Study the drawing (mm; zero at the part's minimum x, y, z) and answer. A direction names the side the tool comes from. Round coordinates to 2 decimals unless told otherwise and drop trailing zeros. Write each loop counter-clockwise with the first axis right and the second up, starting at its lowest first coordinate (ties: lowest second). Pieces come first, ordered by that corner, then holes. Notation, with made-up numbers: (9.5, -15.5) -> (41.5, -15.5) arc R17 ccw to (41.5, 3.5) -> close; hole circle Ø7 at (75, -15.5). An arc over 180 degrees is marked (long way). Return JSON: item names as keys, results as strings.
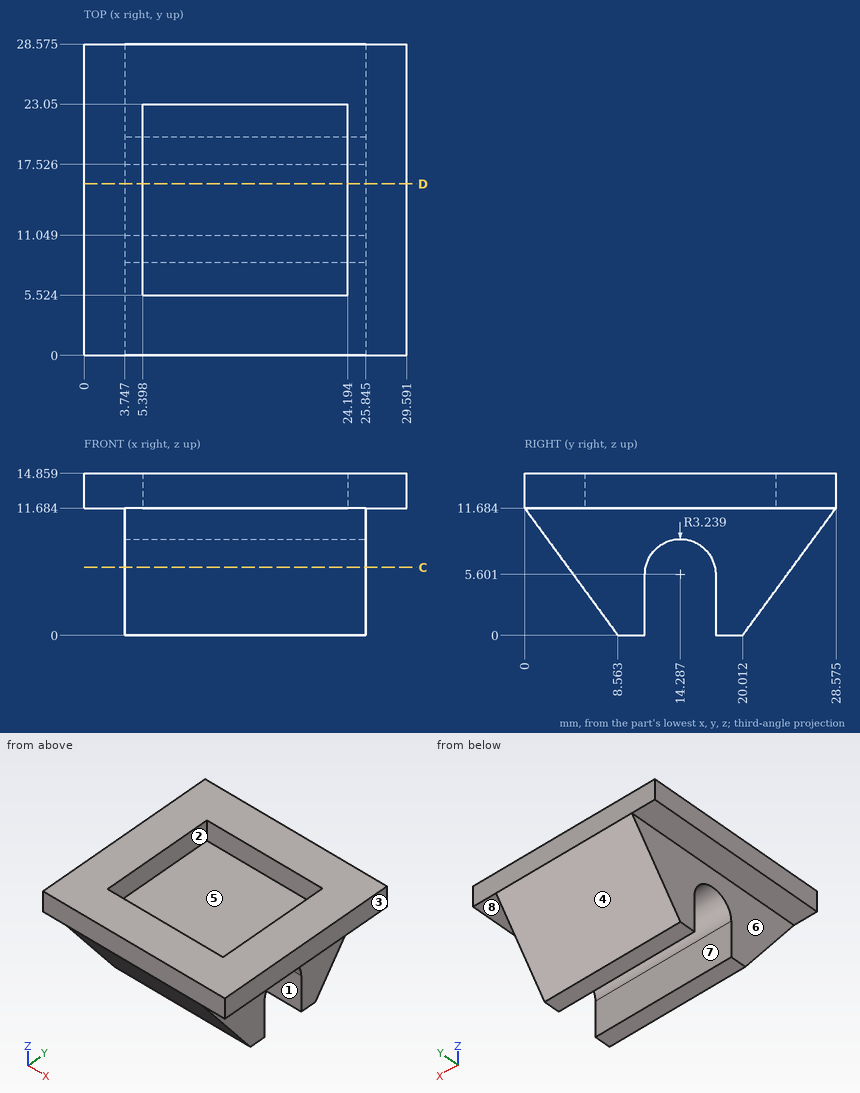
Item 1: Section C-C (z = 6.25) is taken. Give the vertices of the cut face in (x, y) (1 decimal).
Worked answers:
{"outline": "(3.7, 4) -> (25.8, 4) -> (25.8, 11.1) -> (3.7, 11.1) -> close; (3.7, 17.5) -> (25.8, 17.5) -> (25.8, 24.6) -> (3.7, 24.6) -> close"}
Item 2: Straight lines are drawn through the part: L1, parallel to X at y = 3.75, z = 8.75 (1 decimal); L2, parallel to Z at x = 27, y = 21.75 (1 decimal); L3, parallel to X at y = 8, z = 12.5. For each, find the intervals that lie inside material, in ascending order. Write a range as [from, to].
Worked answers:
{"L1": "x = [3.7, 25.8]", "L2": "z = [11.7, 14.9]", "L3": "x = [0, 5.4], [24.19, 29.59]"}
Item 3: A tool of negligible diameter and unlimited length cuts with its end or side. For the marked faces 4, 5, 6, 7 and 8, from which of +Z, -Z, +X, -X, +Y, -Y can it reach the whole face along a straight path? Write none if from no direction.
Worked answers:
{"face 4": "-Z, +X, -X, +Y", "face 5": "+Z", "face 6": "-Z, -X, +Y, -Y", "face 7": "-Z, +X, -X", "face 8": "-Z, +X, +Y, -Y"}
Item 4: Flat-ended cylindrical pins translate along their axes: pin 1 (3 mm diameter, centred on y = 3.5, z = 8.5, fed in from -X); pin 2 (2 mm diameter, centred on x = 7, y = 23, fed in from -Z) (1 decimal); pin 3 (3 mm diameter, centred on x = 20, z = 2.5, fed in from +Y) (1 decimal). Find the tip coordinate at first contact, or state that the pin passes through.
Worked answers:
{"pin 1": "stops at x = 3.75", "pin 2": "stops at z = 2.7", "pin 3": "stops at y = 22.9"}
Item 5: For a pull along X with two mould halves and no side action, classify the marked faces 1, 2 and 3 as released by +X, released by -X, zero draft, split by the parting line, or undercut.
Worked answers:
{"face 1": "zero draft", "face 2": "undercut", "face 3": "released by +X"}
Item 6: Section D-D (y = 15.75) is taken. Give the vertices of the cut face in (x, z) (1 decimal), then the cut area to 3 significant figures.
Worked answers:
{"outline": "(0, 11.7) -> (3.7, 11.7) -> (3.7, 8.5) -> (25.8, 8.5) -> (25.8, 11.7) -> (29.6, 11.7) -> (29.6, 14.9) -> (24.2, 14.9) -> (24.2, 11.7) -> (5.4, 11.7) -> (5.4, 14.9) -> (0, 14.9) -> close", "area": "105 mm2"}
